Autodesk Fusion 360 part; units mm, degrees
sketch "Sketch1" plane through (0, 0, 0) normal (0, 0, 1) x (1, 0, 0)
  line L0 (0, 0) -> (115.84, 0)
  line L1 (115.84, 0) -> (115.84, 117)
  line L2 (115.84, 117) -> (0, 117)
  line L3 (0, 117) -> (0, 0)
  line L4 (10, 7) -> (105.84, 7)
  line L5 (105.84, 7) -> (105.84, 112)
  line L6 (105.84, 112) -> (10, 112)
  line L7 (10, 112) -> (10, 7)
  line L8 (10, 67) -> (105.84, 67)
  line L9 (105.84, 67) -> (105.84, 62)
  line L10 (105.84, 62) -> (10, 62)
  line L11 (10, 62) -> (10, 67)
  circle A0 centre (5, 112) radius 2.75
  circle A1 centre (5, 5) radius 2.75
  circle A2 centre (110.84, 5) radius 2.75
  circle A3 centre (110.84, 112) radius 2.75
  circle A4 centre (5, 112) radius 1.6
  circle A5 centre (5, 5) radius 1.6
  circle A6 centre (110.84, 5) radius 1.6
  circle A7 centre (110.84, 112) radius 1.6
  dimension "d1" = 115.84
  dimension "d2" = 117
  dimension "d3" = 95.84
  dimension "d4" = 105
  dimension "d5" = 5
  dimension "d6" = 10
  dimension "d7" = 5
  dimension "d8" = 55
  dimension "d43" = 5.5
  dimension "d44" = 5
  dimension "d45" = 5
  dimension "d46" = 5.5
  dimension "d47" = 5
  dimension "d48" = 5
  dimension "d49" = 5.5
  dimension "d50" = 5
  dimension "d51" = 5
  dimension "d52" = 5.5
  dimension "d53" = 5
  dimension "d54" = 5
  dimension "d88" = 3.2
  dimension "d89" = 3.2
  dimension "d90" = 3.2
  dimension "d91" = 3.2
extrude "Extrude1" add sketch "Sketch1" against normal blind 78.85 contours L0 L1 L2 L3 | L4 L5 L7 L10 | L5 L7 L8 L9 L10 L11 | L5 L6 L7 L8 | A0 | A1 | A2 | A3 | A4 | A5 | A6 | A7
extrude "Extrude2" cut sketch "Sketch1" against normal blind 73.85 contours L4 L5 L7 L10 | L5 L6 L7 L8
extrude "Extrude7" cut sketch "Sketch1" against normal blind 5 contours A0 | A1 | A2 | A3 | A4 | A5 | A6 | A7
extrude "Extrude11" cut sketch "Sketch1" against normal blind 25 contours A4 | A5 | A6 | A7
ref_plane "WorkPlane1" through (0, 30, 0) normal (0, 1, 0) x (0, 0, 1)
sketch "Sketch2" plane through (0, 30, 0) normal (0, 1, 0) x (1, 0, 0)
  line L0 (10, 48.425) -> (20, 48.425)
  line L1 (20, 48.425) -> (20, 25.425)
  line L2 (20, 25.425) -> (10, 25.425)
  line L3 (10, 25.425) -> (10, 48.425)
  line L4 (115.84, 0) -> (0, 0)
  line L5 (105.84, 25.425) -> (90.84, 25.425)
  line L6 (90.84, 25.425) -> (90.84, 48.425)
  line L7 (90.84, 48.425) -> (105.84, 48.425)
  line L8 (105.84, 48.425) -> (105.84, 25.425)
  line L9 (0, 0) -> (0, 78.85)
  line L10 (115.84, 0) -> (115.84, 78.85)
  dimension "d14" = 10
  dimension "d15" = 23
  dimension "d16" = 25.425
  dimension "d17" = 15
  dimension "d18" = 23
  dimension "d19" = 25.425
  dimension "d20" = 10
  dimension "d21" = 10
extrude "Extrude3" cut sketch "Sketch2" along normal blind 60
ref_plane "WorkPlane2" through (125.84, 58.5, -39.425) normal (1, 0, 0) x (0, -1, 0)
sketch "Sketch3" plane through (125.84, 0, 0) normal (1, 0, 0) x (0, 0, -1)
  line L0 (31.925, 27) -> (41.925, 27)
  line L1 (41.925, 27) -> (41.925, 7)
  line L2 (41.925, 7) -> (31.925, 7)
  line L3 (31.925, 7) -> (31.925, 27)
  line L4 (0, 0) -> (78.85, 0)
  line L5 (0, 0) -> (0, 117)
  dimension "d25" = 10
  dimension "d26" = 20
  dimension "d27" = 7
  dimension "d28" = 31.925
extrude "Extrude4" cut sketch "Sketch3" against normal blind 160
fillet "Fillet1" radius 5 4 edges at (115.84, 117, -39.425) (0, 117, -39.425) (115.84, 0, -39.425) (0, 0, -39.425)
ref_plane "WorkPlane3" through (0, 70, 0) normal (0, 1, 0) x (0, 0, 1)
sketch "Sketch4" plane through (0, 70, 0) normal (0, 1, 0) x (1, 0, 0)
  line L0 (30.42, 56.925) -> (85.42, 56.925)
  line L1 (85.42, 56.925) -> (85.42, 21.925)
  line L2 (85.42, 21.925) -> (30.42, 21.925)
  line L3 (30.42, 21.925) -> (30.42, 56.925)
  line L4 (40.42, 51.925) -> (75.42, 51.925)
  line L5 (75.42, 51.925) -> (75.42, 26.925)
  line L6 (75.42, 26.925) -> (40.42, 26.925)
  line L7 (40.42, 26.925) -> (40.42, 51.925)
  circle A0 centre (35.42, 51.925) radius 2.75
  circle A1 centre (35.42, 26.925) radius 2.75
  circle A2 centre (80.42, 51.925) radius 2.75
  circle A3 centre (80.42, 26.925) radius 2.75
  line L8 (115.84, 0) -> (0, 0)
  line L9 (115.84, 0) -> (115.84, 78.85)
  circle A4 centre (35.42, 26.925) radius 1.6
  circle A5 centre (35.42, 51.925) radius 1.6
  circle A6 centre (80.42, 51.925) radius 1.6
  circle A7 centre (80.42, 26.925) radius 1.6
  dimension "d58" = 55
  dimension "d59" = 35
  dimension "d60" = 35
  dimension "d61" = 25
  dimension "d62" = 10
  dimension "d63" = 5
  dimension "d64" = 5.5
  dimension "d65" = 5
  dimension "d66" = 5
  dimension "d67" = 5.5
  dimension "d68" = 5
  dimension "d69" = 5
  dimension "d70" = 5.5
  dimension "d71" = 5
  dimension "d72" = 5
  dimension "d73" = 5.5
  dimension "d74" = 5
  dimension "d75" = 5
  dimension "d76" = 21.925
  dimension "d77" = 30.42
  dimension "d82" = 3.2
  dimension "d83" = 3.2
  dimension "d84" = 3.2
  dimension "d85" = 3.2
extrude "Extrude8" cut sketch "Sketch4" against normal blind 15 contours L4 L5 L6 L7
extrude "Extrude9" cut sketch "Sketch4" against normal blind 7 contours A0 | A1 | A2 | A3 | A4 | A5 | A6 | A7
extrude "Extrude10" cut sketch "Sketch4" against normal blind 15 contours A4 | A5 | A6 | A7
fillet "Fillet5" radius 6 8 edges at (57.92, 0, -78.85) (114.3755, 1.4645, -78.85) (115.84, 58.5, -78.85) (114.3755, 115.5355, -78.85) (57.92, 117, -78.85) (1.4645, 115.5355, -78.85) (0, 58.5, -78.85) (1.4645, 1.4645, -78.85)
Design review of the part built by this model. Coordinates are the model's own, in mm. A direction names the side the tool comes from. Coordinates: 2 decimals unless noted, no trailing zeros. Loops run counter-clockwise (first coordinate to the right, second up) from the corner with the lowest first, then second, coordinate; pieces in that order, holes last. Notation, with made-up numbers: (84, -20.5) - (125, -20.5) arc R12 ccw to (125, -3.5) - close; hole circle Ø4 at (37.25, 39). An arc over 180 degrees is marked (long way). Use CSV: the item, a comma, the result in double quotes. Start each with the question number.
1. Add section C-C on z = -12. Give the boundary of the cut face in (x, y), plus the area to 3 significant figures.
2. Add section A-A on x = 80.42. Count the separate pieces of the cut face and the enclosed holes in it, plus the area to 3 significant figures.
3. Add section B-B on y = 16. Give the boundary of the cut face in (x, z) (3 decimals), plus the area to 3 significant figures.
4. For faces 1 (the flat face through (113, 5, -5)), 2 (the flat face through (82, 63, -26)), 3 (the flat face through (111, 17, -41.925)), list the 3-axis set-ups (+Z, -Z, +X, -X, +Y, -Y) from which the entire face can be reached by the end or side of a thin tool; tool diameter is ignored.
5. To check wall thickness, follow probe 1 along Y at (x, z) = (48.5, -62.5); probe 2 along Y at (x, z) = (110.84, -19.75); probe 3 along Z at (x, y) = (80.42, 62.7) (3 decimals). State the ranges of each line that lie inside material, in increasing order.
6. Clearance check with flat-ended pins moving along their axes: pin 1 (8 mm diameter, centred on x = 27, y = 22, fed in from +Z); pin 2 (3.5 mm diameter, centred on x = 5, y = 112, fed in from +Z). State where each tip first meets the part, or that it passes through.
7. Add section D-D on x = 97. Give the boundary of the cut face in (y, z) (3 decimals), plus the area to 3 significant figures.
8. Mouldability with a two-part tool opening along X and no side actions: class faces 4 (the flat face through (10, 60, -36)), 5 (the flat face through (58, 63, 0)) as released by +X, released by -X, zero draft, split by the parting line, or undercut.
Resolved:
1,outline,"(0, 5) arc R5 ccw to (5, 0) - (110.84, 0) arc R5 ccw to (115.84, 5) - (115.84, 112) arc R5 ccw to (110.84, 117) - (5, 117) arc R5 ccw to (0, 112) - close; hole circle Ø3.2 at (5, 5); hole circle Ø3.2 at (5, 112); hole (10, 7) - (105.84, 7) - (105.84, 62) - (10, 62) - close; hole (10, 67) - (105.84, 67) - (105.84, 112) - (10, 112) - close; hole circle Ø3.2 at (110.84, 5); hole circle Ø3.2 at (110.84, 112)"
1,area,"3,920 mm2"
2,separate pieces,"3"
2,enclosed holes,"0"
2,area,"1,770 mm2"
3,outline,"(0, -72.85) arc R6 ccw to (6, -78.85) - (109.84, -78.85) arc R6 ccw to (115.84, -72.85) - (115.84, -41.925) - (105.84, -41.925) - (105.84, -73.85) - (10, -73.85) - (10, -41.925) - (0, -41.925) - close; (0, -31.925) - (10, -31.925) - (10, 0) - (0, 0) - close; (105.84, -31.925) - (115.84, -31.925) - (115.84, 0) - (105.84, 0) - close"
3,area,"1,840 mm2"
4,face 1,"+Z"
4,face 2,"none"
4,face 3,"+X, -X"
5,probe 1,"0 to 7, 62 to 67, 112 to 117"
5,probe 2,"0 to 3.4, 6.6 to 110.4, 113.6 to 117"
5,probe 3,"-78.85 to -53.525, -50.325 to -28.525, -25.325 to 0"
6,pin 1,"z = -73.85"
6,pin 2,"z = -5"
7,outline,"(0, -72.85) arc R6 ccw to (6, -78.85) - (111, -78.85) arc R6 ccw to (117, -72.85) - (117, 0) - (112, 0) - (112, -73.85) - (67, -73.85) - (67, -48.425) - (62, -48.425) - (62, -73.85) - (7, -73.85) - (7, 0) - (0, 0) - close; (62, -25.425) - (67, -25.425) - (67, 0) - (62, 0) - close"
7,area,"1,710 mm2"
8,face 4,"undercut"
8,face 5,"zero draft"
